For this review, take the finished solid that the model builds, in its own axes (mm). A direction names the side the tool comes from. Coordinates: 2 decimals unless noted, no trailing zeros. Loops run counter-clockwise (first coordinate to the right, second up) from the corner with the lowest first, then second, coordinate; pieces in that order, holes last. Notation, with made-up numbers: (46, -12) - (96, -12) arc R18 ccw to (96, 15) - close; hole circle Ø3 at (-0.75, 36). An arc over 180 degrees is marked (long way). One line per item, written item: value. Start each with the question number.
1. To check wall thickness, follow line 1 (Z direction, x = -3.25, y = -0.25); line 2 (Y direction, x = 1.25, z = -3.5); line 3 (Z direction, x = 0, y = -2.5). State the ranges of each line that lie inside material, in increasing order. Write a range as from..to.
2. Insertion check: pin 1 (1.5 mm diameter, centred on x = -0.5, z = -45, fed in from -Y); pin 2 (0.7 mm diameter, centred on y = 0, z = 1, fed in from +X); pin 3 (1.5 mm diameter, centred on y = -1.5, z = -17, fed in from +X). Each pin has a flat end and moves straight along its axis. Give the tip position at first contact, or say it passes through.
3. Take a section at A-A, the plane z = -6.5. State the section outline as (x, y) points.
4. For faces 1 (the face through (2, 0, 2.3)), 2 (the face through (-0.616, -1.088, 1.413)), 3 (the face through (0, -2, -45)), list the 3-axis set-ups (+Z, -Z, +X, -X, +Y, -Y) from which the entire face can be reached by the end or side of a thin tool; tool diameter is ignored.
Solid Edge part; units mm, degrees
sketch "Sketch1" plane through (0, 0, 0) normal (0, -1, 0) x (1, 0, 0)
  line L0 (2, 0) -> (4, 2)
  line L1 (4, 2) -> (4, 2.3)
  line L2 (4, 2.3) -> (0, 2.3)
  line L3 (0, 2.3) -> (0, -57.7)
  line L4 (0, -57.7) -> (1.5705, -57.7)
  line L5 (1.5705, -57.7) -> (2, -57.2705)
  line L6 (2, -57.2705) -> (2, -33.7)
  line L7 (2, -33.7) -> (1.5705, -33.7)
  line L8 (1.5705, -33.7) -> (1.5705, -33.69)
  line L9 (1.5705, -33.69) -> (2, -33.69)
  line L10 (2, -33.69) -> (2, 0)
  dimension "D1" = 2
  dimension "D2" = 1.5705
revolve "RevolvedProtrusion1" add sketch "Sketch1" angle 360 about axis through (0, 0, 54) along (0, 0, -1)
sketch "Sketch2" plane through (0, 0, 0) normal (0, -1, 0) x (1, 0, 0)
  arc A0 (-1.25, 0.5) -> (0, 0) centre (0, 1.8125) ccw
  line L0 (0, 0.5) -> (0, 0)
  line L1 (-1.25, 0.5) -> (0, 0.5)
revolve "RevolvedCutout1" cut sketch "Sketch2" angle 360 about axis through (0, 0, 54) along (0, 0, -1)
sketch "Sketch3" plane through (0, 0, 2.3) normal (0, 0, 1) x (0, -1, 0)
  line L0 (-1.4434, 0) -> (-0.7217, 1.25)
  line L1 (-0.7217, 1.25) -> (0.7217, 1.25)
  line L2 (0.7217, 1.25) -> (1.4434, 0)
  line L3 (1.4434, 0) -> (0.7217, -1.25)
  line L4 (0.7217, -1.25) -> (-0.7217, -1.25)
  line L5 (-0.7217, -1.25) -> (-1.4434, 0)
extrude "Cutout1" cut sketch "Sketch3" against normal blind 1.8
cosmetic_thread "Thread1"
sketch "Sketch4" plane through (0, 0, 0) normal (1, 0, 0) x (0, 1, 0)
  line L0 (-1.435, 2.3) -> (0, 1.4715)
revolve "RevolvedCutout2" cut sketch "Sketch4" angle 360 about axis through (0, 0, -57) along (0, 0, 1) material side at (0, -0.6925, 1.9291)
fillet "Round1" radius 0.2 1 edges at (-2, 0, 0)
properties material "Stahl"
Solutions:
1. line 1: 1.26..2.3
1. line 2: -1.56..1.56
1. line 3: 0.5..2.3
2. pin 1: y = -2
2. pin 2: x = 3.35
2. pin 3: x = 1.85
3. outline: circle Ø4 at (0, 0)
4. face 1: +Z, +X, -X, +Y, -Y
4. face 2: +Z
4. face 3: -Z
